from build123d import *

# Parameters (mm, degrees)
SKETCH1_R               = 9.75
BOSS_EXTRUDE1_DEPTH     = 18
SKETCH4_5_R             = 1.5
SKETCH4_5_R_2           = 1.6
BOSS_EXTRUDE3_DEPTH     = 3
BOSS_EXTRUDE5_REACH     = 41.383
SKETCH1_4_R             = 7.5
CUT_EXTRUDE2_DEPTH      = 9
CUT_EXTRUDE8_START      = 18
SKETCH1_6_R             = 8.05
CUT_EXTRUDE8_DEPTH      = 6.5
CUT_EXTRUDE5_DEPTH      = 40.383499083
CUT_EXTRUDE5_DEPTH_BACK = 40.383499083
SKETCH4_R               = 1.6
FILLET8_R               = 11
FILLET9_R               = 3
CUT_EXTRUDE9_START      = 11.5
SKETCH1_8_R             = 5
CUT_EXTRUDE9_DEPTH      = 4
BOSS_EXTRUDE6_REACH     = 41.383
SKETCH5_R               = 1.6


# Some blends are built 0.0001 mm under size
with BuildPart() as part:
    # Sketch1 → Boss-Extrude1 (new body)
    with BuildSketch(Plane(origin=(0, 0, 0), x_dir=(1, 0, 0), z_dir=(0, 1, 0))):
        with Locations(Location((0, 0, 0), (0, 0, 270))):
            Circle(SKETCH1_R)
    extrude(amount=BOSS_EXTRUDE1_DEPTH)

    # Sketch4<5> → Boss-Extrude3 (add)
    with BuildSketch(Plane(origin=(0, 0, -9.75), x_dir=(-1, 0, 0), z_dir=(0, 0, -1))):
        Polygon((-9.75, 18), (-9.75, 6), (-29.1, 6), (-29.1, 0), (9.75, 0), (9.75, 18), align=None)
        with Locations((-26.1, 3)):
            Circle(SKETCH4_5_R, mode=Mode.SUBTRACT)
        with Locations((0, 3)):
            Circle(SKETCH4_5_R_2, mode=Mode.SUBTRACT)
    extrude(amount=-BOSS_EXTRUDE3_DEPTH)

    # Sketch4<8> → Boss-Extrude5 (add, up to next)
    with BuildSketch(Plane(origin=(0, 0, -9.75), x_dir=(-1, 0, 0), z_dir=(0, 0, -1)), mode=Mode.PRIVATE) as boss_extrude5_sk1:
        with BuildLine():
            Line((0, 18), (-9.75, 18))
            Line((-9.75, 18), (-9.75, 6))
            Line((-9.75, 6), (-9.75, 0))
            Line((-9.75, 0), (0, 0))
            Line((0, 0), (0, 1.4))
            ThreePointArc((0, 1.4), (-1.6, 3), (0, 4.6))
            Line((0, 4.6), (0, 18))
        make_face()
    boss_extrude5_tool1 = extrude(boss_extrude5_sk1.sketch, amount=-BOSS_EXTRUDE5_REACH, mode=Mode.PRIVATE) - part.part
    # Sketch4<8> → Boss-Extrude5 (add, up to next)
    with BuildSketch(Plane(origin=(0, 0, -9.75), x_dir=(-1, 0, 0), z_dir=(0, 0, -1)), mode=Mode.PRIVATE) as boss_extrude5_sk2:
        with BuildLine():
            Line((9.75, 18), (0, 18))
            Line((0, 18), (0, 4.6))
            ThreePointArc((0, 4.6), (1.13137085, 4.13137085), (1.6, 3))
            ThreePointArc((1.6, 3), (1.13137085, 1.86862915), (0, 1.4))
            Line((0, 1.4), (0, 0))
            Line((0, 0), (9.75, 0))
            Line((9.75, 0), (9.75, 18))
        make_face()
    boss_extrude5_tool2 = extrude(boss_extrude5_sk2.sketch, amount=-BOSS_EXTRUDE5_REACH, mode=Mode.PRIVATE) - part.part
    add(boss_extrude5_tool1.solids().sort_by_distance((4.973396, 9.140702, -9.75))[0])
    add(boss_extrude5_tool2.solids().sort_by_distance((-4.973396, 9.140702, -9.75))[0])

    # Sketch1<4> → Cut-Extrude2 (cut)
    with BuildSketch(Plane(origin=(0, 0, 0), x_dir=(1, 0, 0), z_dir=(0, 1, 0))):
        with Locations(Location((0, 0, 0), (0, 0, 270))):
            Circle(SKETCH1_4_R)
    extrude(amount=CUT_EXTRUDE2_DEPTH, mode=Mode.SUBTRACT)

    # Sketch1<6> → Cut-Extrude8 (cut)
    with BuildSketch(Plane(origin=(0, 0, 0), x_dir=(1, 0, 0), z_dir=(0, 1, 0)).offset(CUT_EXTRUDE8_START)):
        with Locations(Location((0, 0, 0), (0, 0, 270))):
            Circle(SKETCH1_6_R)
    extrude(amount=-CUT_EXTRUDE8_DEPTH, mode=Mode.SUBTRACT)

    # Sketch4 → Cut-Extrude5 (cut, two sides: drawn at the far end of the back side and taken through both)
    with BuildSketch(Plane(origin=(0, 0, -9.75), x_dir=(-1, 0, 0), z_dir=(0, 0, -1)).offset(-CUT_EXTRUDE5_DEPTH_BACK)):
        with Locations((0, 3)):
            Circle(SKETCH4_R)
    extrude(amount=CUT_EXTRUDE5_DEPTH + CUT_EXTRUDE5_DEPTH_BACK, mode=Mode.SUBTRACT)

    # Fillet8
    # the kernel refuses this fillet: 11 mm, written as the material it adds along each edge
    with BuildSketch(Plane(origin=(9.75, 0, -6.75), x_dir=(1, 0, 0), z_dir=(0, 1, 0))) as fillet8_piece_1:
        with BuildLine():
            CenterArc((10.560096012, -11), FILLET8_R, 90, 78.18108009)
            Line((-0.206701874, -8.746987952), (-1.283381663, -8.521686747))
            ThreePointArc((-1.283381663, -8.521686747), (-1.1, -6.75), (-1.1, 0))
            Line((-1.1, 0), (0, 1.1))
            Line((0, 1.1), (10.560096012, 1.1))
            Line((10.560096012, 1.1), (10.560096012, 0))
        make_face()
    extrude(amount=6)

    # Fillet9
    fillet9_edges = [part.edges().sort_by_distance(p)[0] for p in [
        (29.1, 0, -8.25),
        (29.1, 6, -8.25),
    ]]
    fillet(fillet9_edges, radius=FILLET9_R - 0.0001)  # a hair under: the kernel refuses the full size

    # Sketch1<8> → Cut-Extrude9 (cut)
    with BuildSketch(Plane(origin=(0, 0, 0), x_dir=(1, 0, 0), z_dir=(0, 1, 0)).offset(CUT_EXTRUDE9_START)):
        with Locations(Location((0, 0, 0), (0, 0, 270))):
            Circle(SKETCH1_8_R)
    extrude(amount=-CUT_EXTRUDE9_DEPTH, mode=Mode.SUBTRACT)

    # Sketch5 → Boss-Extrude6 (add, up to next)
    with BuildSketch(Plane.XY.offset(9.75), mode=Mode.PRIVATE) as boss_extrude6_sk1:
        Polygon((9.75, 0), (-9.75, 0), (-9.75, 18), (9.75, 18), (9.75, 6), align=None)
        with Locations(Location((0, 3, 0), (0, 0, 180))):
            Circle(SKETCH5_R, mode=Mode.SUBTRACT)
    boss_extrude6_tool1 = extrude(boss_extrude6_sk1.sketch, amount=-BOSS_EXTRUDE6_REACH, mode=Mode.PRIVATE) - part.part
    add(boss_extrude6_tool1.solids().sort_by_distance((0, 9.140702, 9.75))[0])
    add(boss_extrude6_tool1.solids().sort_by_distance((0, 9.140702, 9.75))[1])


solid = part.part
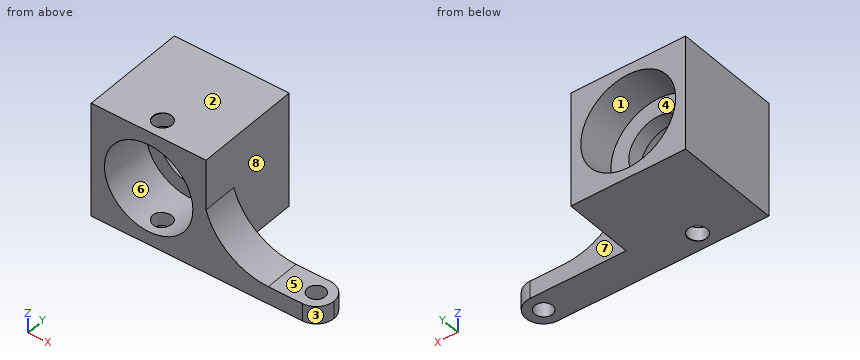
Source: CAD feature listing. Evaluate the final solid. Frame: model axes, mm. Face numbers are marked on the shaded views. A direction names the side the tool comes from. Give positions to 0.01 mm unless a question says otherwise; leave off trailing zeros. Write each loop counter-clockwise with the first axis right and the second up, starting at its lowest first coordinate (ties: lowest second). Pieces come first, ordered by that corner, then holes. Notation, with made-up numbers: (-38.75, 31) -> (10.25, 31) arc R18 cw to (10.25, 47) -> close; hole circle Ø8 at (28, -29.75). An arc over 180 degrees is marked (long way). Write item = value, one per line.
Q1. First-contact query: pin 1 (5.5 mm diameter, centred on y = 5.5, z = -1, fed in from +X); pin 2 (4.5 mm diameter, centred on x = 3.5, z = 1.5, fed in from -Y); pin 3 (3 mm diameter, centred on x = 0, y = 3, fed in from +Z); pin 4 (1.5 mm diameter, centred on x = 14, y = 2.5, fed in from +Z). Flat tips, straight axial feed; report the tip coordinate or a pass-through.
Here are the results:
pin_1 = 12.76
pin_2 = 9
pin_3 = through
pin_4 = -4.19
Q2. Cut plane A-A on z = 0. Return loops of the section in (x, y), then the cut area to 3 significant figures.
Here are the results:
outline = (-9.75, 0) -> (-7.5, 0) -> (-7.5, 9) -> (-5, 9) -> (-5, 11.5) -> (-8.05, 11.5) -> (-8.05, 18) -> (-9.75, 18) -> close; (5, 9) -> (7.5, 9) -> (7.5, 0) -> (10.16, 0) -> (10.16, 6) -> (9.75, 6) -> (9.75, 18) -> (8.05, 18) -> (8.05, 11.5) -> (5, 11.5) -> close
area = 88.8 mm²
Q3. Mould query, pull axis X, two halves, no side actions, for the marked faces 1, 2, 3 and 4. Classes: +X half, -X half, draft (parallel to the pull), parting line (faces both ways), or undercut.
Here are the results:
face_1 = undercut
face_2 = draft
face_3 = +X half
face_4 = undercut
Q4. Reachability of the marked faces 5, 6, 7 and 8 from +Z, -Z, +X, -X, +Y, -Y: full face, straight path, thin tool, end or side. Return the list, or none.
Here are the results:
face_5 = +Z, +X, +Y, -Y
face_6 = -Y
face_7 = +Z, -Z, +X, +Y
face_8 = +Z, +X, +Y
Q5. Line query: line 1 (Y direction, x = 0, z = 7.95); line 2 (X direction, y = 14.75, z = 0); line 3 (Y direction, x = 26.1, z = -7.85). Output: solid intervals per line, ascending. Write a range as from..to.
Here are the results:
line_1 = 0..1.4, 4.6..11.5
line_2 = -9.75..-8.05, 8.05..9.75
line_3 = 0..1.5, 4.5..6
Q6. Cut plane D-D on y = 8.25. Return loops of the section in (x, z).
Here are the results:
outline = (-9.75, -9.75) -> (9.75, -9.75) -> (9.75, 9.75) -> (-9.75, 9.75) -> close; hole circle Ø15 at (0, 0)
Q7. Cut plane B-B on x = 2. Return loops of the section in (y, z).
Here are the results:
outline = (0, -9.75) -> (18, -9.75) -> (18, -7.8) -> (11.5, -7.8) -> (11.5, -4.58) -> (9, -4.58) -> (9, -7.23) -> (0, -7.23) -> close; (0, 7.23) -> (9, 7.23) -> (9, 4.58) -> (11.5, 4.58) -> (11.5, 7.8) -> (18, 7.8) -> (18, 9.75) -> (0, 9.75) -> close
Q8. Cut plane C-C on y = 13. Return loops of the section in (x, z), then the cut area to 3 significant figures.
Here are the results:
outline = (-9.75, -9.75) -> (9.75, -9.75) -> (9.75, 9.75) -> (-9.75, 9.75) -> close; hole circle Ø16.1 at (0, 0)
area = 177 mm²
